Input: dimensioned drawing with shaded views. Units: mm. Origin: part minimum x, y, z. A direction names the side the tool comes from. Give positions to 0.01 mm unless a question says otherwise; leave off trailing zeros. Loops run counter-clockwise (first coordinate to the right, second up) from the corner with the lowest first, then second, coordinate; pieces in that order, holes last. Notation, with made-up numbers: (9, 54.5) -> (17, 54.5) arc R25 cw to (17, 71.5) -> close; hole circle Ø9 at (-36.75, 32.25). An arc over 180 degrees is marked (long way). Answer in a Markdown table with one row per item. Add a question column.
1) Section query B-B (z = 3.75). Return the cut outline in (x, y) (1 decimal), plus the area to 3 significant figures.
2) Access query for the marked faces 5, 6 and 7. Directions: +Z, -Z, +X, -X, +Y, -Y. A direction counts if a zero-diameter tool reaches every point of the face in a straight line with its end or side. Return the directions, or none.
3) Draft query along Y for the marked faces 1, 2, 3 and 4. Return one class per face: +Y half, -Y half, draft (parallel to the pull), parting line (faces both ways), or undercut.
4) First-contact query: P1, Ø2.5, axis at y = 78.99, z = 3.99, coming from the +X side; P2, Ø1.5, axis at x = 0.5, y = 49, coming from the +Z side (1 decimal); P3, Ø1.5, axis at x = 2, z = 1.5, coming from the -Y side. Flat tips, straight axial feed; report the tip coordinate or a pass-through.
5) Section query A-A (x = 2.9). Return the cut outline in (y, z) (1 decimal), plus the area to 3 significant figures.
6) Section query C-C (y = 39.5). Return the cut outline in (x, z) (1 decimal), plus the area to 3 significant figures.
7) Line query: line 1 (Y direction, x = 1.65, z = 4) (1 decimal); line 2 (Y direction, x = 3.2, z = 4.75) (1 decimal); line 3 (Z direction, x = 3.75, y = 42) (1 decimal). Output: solid intervals per line, ascending. Write a range as from..to.
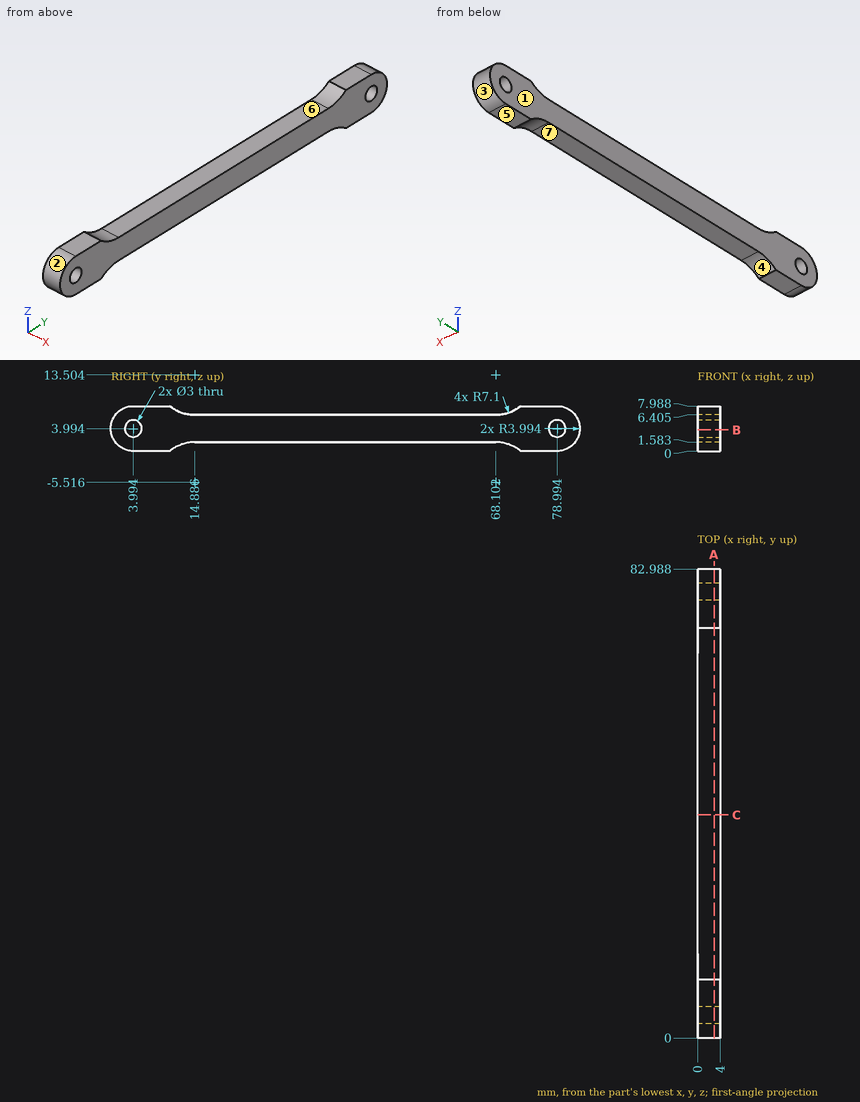
Evaluation:
| question | item | result |
|---|---|---|
| 1 | outline | (0, 0) -> (4, 0) -> (4, 2.5) -> (0, 2.5) -> close; (0, 5.5) -> (4, 5.5) -> (4, 77.5) -> (0, 77.5) -> close; (0, 80.5) -> (4, 80.5) -> (4, 83) -> (0, 83) -> close |
| 1 | area | 308 mm² |
| 2 | face 5 | -Z, +X, -X, +Y, -Y |
| 2 | face 6 | +Z, +X, -X |
| 2 | face 7 | -Z, +X, -X |
| 3 | face 1 | draft |
| 3 | face 2 | -Y half |
| 3 | face 3 | +Y half |
| 3 | face 4 | undercut |
| 4 | P1 | through |
| 4 | P2 | z = 6.4 |
| 4 | P3 | y = 0.4 |
| 5 | outline | (4, 0) -> (10.4, 0) arc R7.1 cw to (14.9, 1.6) -> (68.1, 1.6) arc R7.1 cw to (72.6, 0) -> (79, 0) arc R4 ccw to (79, 8) -> (72.6, 8) arc R7.1 cw to (68.1, 6.4) -> (14.9, 6.4) arc R7.1 cw to (10.4, 8) -> (4, 8) arc R4 ccw to start; hole circle Ø3 at (4, 4); hole circle Ø3 at (79, 4) |
| 5 | area | 447 mm² |
| 6 | outline | (0, 1.6) -> (4, 1.6) -> (4, 6.4) -> (0, 6.4) -> close |
| 6 | area | 19.3 mm² |
| 7 | line 1 | 0..2.5, 5.5..77.5, 80.5..83 |
| 7 | line 2 | 0.1..2.7, 5.3..77.7, 80.3..82.9 |
| 7 | line 3 | 1.6..6.4 |
